from build123d import *

# Parameters (mm, degrees)
F1_DEPTH = 5
F2_R     = 2.5
F3_DEPTH = 6


with BuildPart() as f1:
    # F0 (on Top) → F1 (new body)
    with BuildSketch(Plane.XY):
        Polygon((2.309401, 4), (-2.309401, 4), (-4.618802, 0), (-2.309401, -4), (2.309401, -4), (4.618802, 0), align=None)
    extrude(amount=F1_DEPTH)

    # F2 (on face) → F3 (join)
    with BuildSketch(Plane(origin=(0, 0, 0), x_dir=(1, 0, 0), z_dir=(0, 0, -1))):
        Circle(F2_R)
    extrude(amount=F3_DEPTH)

    # F4 (on Front) → F5 (revolve, cut)
    with BuildSketch(Plane.XZ):
        Polygon((1.241204, 6.975186), (1.241204, 6.27986), (5.267579, 4.024274), (5.267579, 6.975186), align=None)
    revolve(axis=Axis((0, 0, 6.94047), (0, 0, -1)), mode=Mode.SUBTRACT)

    # F6 (on Front) → F7 (revolve)
    with BuildSketch(Plane.XZ):
        with BuildLine():
            Line((0, 6.1), (0, 2.1))
            ThreePointArc((0, 2.1), (2, 4.1), (0, 6.1))
        make_face()
    revolve(axis=Axis((0, 0, 4.1), (0, 0, -1)))


solid = f1.part
Part model, mm, in its own coordinate system. A direction names the side the tool comes from. Coordinates: 2 decimals unless noted, no trailing zeros. Loops run counter-clockwise (first coordinate to the right, second up) from the corner with the lowest first, then second, coordinate; pieces in that order, holes last. Notation, with made-up numbers: (-13, 12.5) -> (27, 12.5) arc R23 cw to (27, 48.5) -> close; hole circle Ø3 at (-22.75, 77). An arc over 180 degrees is marked (long way). Use a Markdown table: item, result. Add a question column.
Item 1: Band-saw the part on B-B on z = 4.25. Write the cut outline in (x, y).
Item 2: Which spindle directions (+Z, -Z, +X, -X, +Y, -Y) get a long thin tool onto all of the face, cutting with end or side? Do faces 1 (the flat face through (-2, 1, 5)), 2 (the flat face through (2, 2, 0)), 3 (the flat face through (0, -4, 2)). Say none if no direction does.
Item 3: Band-saw the part on C-C on z = -3.25. Write the cut outline in (x, y), plus the area to 3 significant figures.
Item 4: Probe probe 1 along Z at (x, y) = (1.5, 3); probe 2 along Z at (x, y) = (-0.25, -2.25); probe 3 along Y at (x, z) = (-4, 2.25). List the from-to ranges inside material, lowest first.
Item 5: Band-saw the part on A-A on x = 0. Write the cut outline in (y, z), plus the area to 3 significant figures.
Item 6: Flat gauge pin, fed straight in: P1, Ø1.5, axis at x = 2, y = 0, coming from the +Z side. Where does the tip first touch, or does it go through?
Geometry says:
| question | item | result |
|---|---|---|
| 1 | outline | (-4.62, 0) -> (-2.31, -4) -> (2.31, -4) -> (4.62, 0) -> (2.31, 4) -> (-2.31, 4) -> close |
| 2 | face 1 | +Z |
| 2 | face 2 | -Z |
| 2 | face 3 | +Z, -Z, +X, -X, -Y |
| 3 | outline | circle Ø5 at (0, 0) |
| 3 | area | 19.6 mm² |
| 4 | probe 1 | 0 to 5 |
| 4 | probe 2 | -6 to 5 |
| 4 | probe 3 | -1.07 to 1.07 |
| 5 | outline | (-4, 0) -> (-2.5, 0) -> (-2.5, -6) -> (2.5, -6) -> (2.5, 0) -> (4, 0) -> (4, 4.73) -> (3.53, 5) -> (1.79, 5) arc R2 ccw to (-1.79, 5) -> (-3.53, 5) -> (-4, 4.73) -> close |
| 5 | area | 72.7 mm² |
| 6 | P1 | z = 5.66 |
